Geometry check sheet. Reference: the model listing, model coordinates, mm. A direction names the side the tool comes from. Give positions to 0.01 mm unless a question says otherwise; leave off trailing zeros. Loops run counter-clockwise (first coordinate to the right, second up) from the corner with the lowest first, then second, coordinate; pieces in that order, holes last.
1. Tool access check on faces 1 (the conical face through (-1.271, -1.251, 26.273)), 2 (the conical face through (-15.903, -0.817, -18.082)), 3 (the flat face through (-74.653, -51.268, 1.122)). Record the directions out of +Z, -Z, +X, -X, +Y, -Y that give a thin tool (end or side, any length) a straight path to the whole face; none if there is none.
2. Material ranges on L1, parallel to Y at x = -57, z = 10; L2, parallel to Y at x = -79, z = -12.5; L3, parallel to X at y = 15, z = -6, recorded low to high.
3. Release check for a two-part mould opening along Y. For faces 4 (the flat face through (2, -17, 30.471)), 5 (the conical face through (-11.733, -0.941, -5.737)), 6 (the conical face through (18, -1.8, -27.2)) record: +Y half, -Y half, draft (parallel to the pull), parting line (faces both ways), or undercut.
4. Cross-section at C-C, the plane z = 13. Record the cut outline in (x, y), plus the area to 3 significant figures.
5. Cross-section at A-A, the plane y = 0. Record the cut outline in (x, z), plus the area to 3 significant figures.
6. Go/stop test with flat-tipped pins: pin 1 Ø6 at (y, z) = (33.5, -7.5) entering from -X; pin 2 Ø8 at (x, y) = (13.5, 26.5) entering from -Z; pin 3 Ø3 at (x, z) = (-30.5, -12.5) entering from -Y; pin 4 Ø2 at (x, z) = (-33, 3) entering from -Y. Record where each tip stops, or that it passes through.
7. Cross-section at B-B, the plane z = -24. Record the cut outline in (x, y), plus the area to 3 significant figures.
from build123d import *

# Parameters (mm, degrees)
F2_ANGLE = 242.631105


with BuildPart() as f2:
    # F0 (on Front) → F2 (revolve, symmetric)
    with BuildSketch(Plane.XZ) as f2_sk:
        Polygon((36.124457, 30.471444), (2.095406, 30.471444), (-1.693323, 26.322305), (5.362239, 25.53685), (-18.062208, -17.349653), (16.651124, -29.059894), (39.228894, 1.446627), align=None)
    revolve(axis=Axis((-43.462213, 0, 5.015243), (0, 0, -1)), revolution_arc=F2_ANGLE / 2)
    revolve(f2_sk.sketch, axis=Axis((-43.462213, 0, 5.015243), (0, 0, 1)), revolution_arc=F2_ANGLE / 2)


solid = f2.part
Result:
1. face 1: none
1. face 2: -Z
1. face 3: +Z, -Z, -X
2. L1: y = -80.65 to -38, 38 to 80.65
2. L2: y = -63.04 to -58.41, 58.41 to 63.04
2. L3: x = -15.65 to 32.25
3. face 4: draft
3. face 5: undercut
3. face 6: parting line
4. outline: (-85.8, -69.59) arc R81.46 ccw (long way) to (-85.8, 69.59) - (-65.28, 35.86) arc R41.98 cw (long way) to (-65.28, -35.86) - close
4. area: 10,300 mm2
5. outline: (-18.06, -17.35) - (16.65, -29.06) - (39.23, 1.45) - (36.12, 30.47) - (2.1, 30.47) - (-1.69, 26.32) - (5.36, 25.54) - close
5. area: 2,220 mm2
6. pin 1: stops at x = -65.67
6. pin 2: stops at z = -29.06
6. pin 3: stops at y = -72.36
6. pin 4: stops at y = -82.02
7. outline: (-76.65, -54.56) arc R63.86 ccw (long way) to (-76.65, 54.56) - (-66.91, 38.54) arc R45.11 cw (long way) to (-66.91, -38.54) - close
7. area: 4,320 mm2
